from build123d import *

# Parameters (mm, degrees)
SKETCH1_W           = 168
SKETCH1_H           = 48
SKETCH1_W_2         = 42
SKETCH1_H_2         = 42
SKETCH1_W_3         = 72
BOSS_EXTRUDE1_DEPTH = 10
SKETCH2_W           = 18
SKETCH2_H           = 10
CUT_EXTRUDE1_DEPTH  = 10
SKETCH3_W           = 42
SKETCH3_H           = 42
SKETCH3_W_2         = 32
SKETCH3_H_2         = 32
BOSS_EXTRUDE2_DEPTH = 7
BOSS_EXTRUDE3_DEPTH = 7
FILLET1_R           = 10
SKETCH6_W           = 18
SKETCH6_H           = 7
BOSS_EXTRUDE4_DEPTH = 3


with BuildPart() as part:
    # Sketch1 → Boss-Extrude1 (new body)
    with BuildSketch(Plane(origin=(0, 0, 0), x_dir=(1, 0, 0), z_dir=(0, 1, 0))):
        with Locations((-81, 21)):
            Rectangle(SKETCH1_W, SKETCH1_H)
        with Locations((-141, 21)):
            Rectangle(SKETCH1_W_2, SKETCH1_H_2, mode=Mode.SUBTRACT)
        with Locations((-21, 21)):
            Rectangle(SKETCH1_W_2, SKETCH1_H_2, mode=Mode.SUBTRACT)
        with Locations((-81, 21)):
            Rectangle(SKETCH1_W_3, SKETCH1_H_2, mode=Mode.SUBTRACT)
    extrude(amount=BOSS_EXTRUDE1_DEPTH)

    # Sketch2 → Cut-Extrude1 (cut)
    with BuildSketch(Plane(origin=(0, 0, -45), x_dir=(-1, 0, 0), z_dir=(0, 0, -1))):
        with Locations((21, 5)):
            Rectangle(SKETCH2_W, SKETCH2_H)
        with Locations((141, 5)):
            Rectangle(SKETCH2_W, SKETCH2_H)
    extrude(amount=-CUT_EXTRUDE1_DEPTH, mode=Mode.SUBTRACT)

    # Sketch3 → Boss-Extrude2 (add)
    with BuildSketch(Plane.XZ):
        with Locations((-21, -21)):
            Rectangle(SKETCH3_W, SKETCH3_H)
        with Locations((-21, -21)):
            Rectangle(SKETCH3_W_2, SKETCH3_H_2, mode=Mode.SUBTRACT)
    extrude(amount=-BOSS_EXTRUDE2_DEPTH)

    # Sketch4 → Boss-Extrude3 (add)
    with BuildSketch(Plane(origin=(0, 10, 0), x_dir=(1, 0, 0), z_dir=(0, 1, 0))):
        Polygon((-42, 42), (-30, 42), (-30, 45), (-42, 45), (-45, 45), (-45, 42), (-45, 0), (-45, -3), (-42, -3), (3, -3), (3, 0), (3, 42), (3, 45), (0, 45), (-12, 45), (-12, 42), (0, 42), (0, 0), (-42, 0), align=None)
    extrude(amount=BOSS_EXTRUDE3_DEPTH)

    # Fillet1
    fillet1_edges = [part.edges().sort_by_distance(p)[0] for p in [
        (-117, 5, -42),
        (-117, 5, 0),
        (-45, 5, 0),
        (-45, 5, -42),
    ]]
    fillet(fillet1_edges, radius=FILLET1_R)

    # Sketch6 → Boss-Extrude4 (add)
    with BuildSketch(Plane(origin=(0, 0, -42), x_dir=(-1, 0, 0), z_dir=(0, 0, -1))):
        with Locations((21, 3.5)):
            Rectangle(SKETCH6_W, SKETCH6_H)
    extrude(amount=BOSS_EXTRUDE4_DEPTH)


solid = part.part
Verification items for the finished model (mm, model axes). A direction names the side the tool comes from. Round coordinates to 2 decimals unless told otherwise and drop trailing zeros. Loops run counter-clockwise (first coordinate to the right, second up) from the corner with the lowest first, then second, coordinate; pieces in that order, holes last. Notation, with made-up numbers: (66, 21.5) - (110, 21.5) arc R6 ccw to (110, 30.5) - close; hole circle Ø5 at (1.25, 39.25). An arc over 180 degrees is marked (long way). Write item = value, one per line.
Q1. Sectioned sample at D-D on z = -39.5. Record the boundary of the cut face in (x, y).
Here are the results:
outline = (-165, 0) - (-162, 0) - (-162, 10) - (-165, 10) - close; (-120, 0) - (-113.61, 0) - (-113.61, 10) - (-120, 10) - close; (-48.39, 0) - (3, 0) - (3, 17) - (0, 17) - (0, 7) - (-42, 7) - (-42, 17) - (-45, 17) - (-45, 10) - (-48.39, 10) - close
Q2. Tool access check on faces 4 (the flat face through (0, 12, -21)), 5 (the flat face through (-30, 12, -43)), 6 (the flat face through (-150, 5, -44)), 7 (the flat face through (-43, 0, -19)), 8 (the flat face through (-21, 3, -37)). Record the directions out of +Z, -Z, +X, -X, +Y, -Y that give a thin tool (end or side, any length) a straight path to the whole face; none if there is none.
Here are the results:
face_4 = +Y
face_5 = -Z, +Y
face_6 = -Z, +Y, -Y
face_7 = +Z, -Z, +X, -X, -Y
face_8 = +Y, -Y
Q3. Sectioned sample at C-C on y = 5.25. Record the boundary of the cut face in (x, z).
Here are the results:
outline = (-165, -45) - (-150, -45) - (-150, -42) - (-162, -42) - (-162, 0) - (-120, 0) - (-120, -42) - (-132, -42) - (-132, -45) - (3, -45) - (3, 3) - (-165, 3) - close; hole (-117, -32) arc R10 ccw to (-107, -42) - (-55, -42) arc R10 ccw to (-45, -32) - (-45, -10) arc R10 ccw to (-55, 0) - (-107, 0) arc R10 ccw to (-117, -10) - close; hole (-37, -37) - (-5, -37) - (-5, -5) - (-37, -5) - close
Q4. Mould release check, pull along X, two halves, no side actions. Record for faces 1 (the flat face through (-64, 6, 3)), 2 (the flat face through (-81, 5, -42)), 3 (the flat face through (3, 8, -21)): +X half, -X half, draft (parallel to the pull), parting line (faces both ways), or undercut.
Here are the results:
face_1 = draft
face_2 = undercut
face_3 = +X half
Q5. Sectioned sample at B-B on x = -25.5. Record the boundary of the cut face in (y, z), plus the area to 3 significant figures.
Here are the results:
outline = (0, -45) - (7, -45) - (7, -37) - (0, -37) - close; (0, -5) - (7, -5) - (7, 0) - (17, 0) - (17, 3) - (0, 3) - close
area = 142 mm^2
Q6. Sectioned sample at A-A on z = -20. Record the boundary of the cut face in (x, y), plus the area to 3 significant figures.
Here are the results:
outline = (-165, 0) - (-162, 0) - (-162, 10) - (-165, 10) - close; (-120, 0) - (-117, 0) - (-117, 10) - (-120, 10) - close; (-45, 0) - (-37, 0) - (-37, 7) - (-42, 7) - (-42, 17) - (-45, 17) - close; (-5, 0) - (3, 0) - (3, 17) - (0, 17) - (0, 7) - (-5, 7) - close
area = 232 mm^2
Q7. Depth check by flat-ended pin: pin 1 (3 mm diameter, centred on x = -149.5, y = 3.5, fed in from -Z). Enter the tip coordinate at first touch or a pass-through.
Here are the results:
pin_1 = -45
Q8. Material ranges on L1, parallel to X at y = 11.75, z = -40.5; L2, parallel to X at y = 1, z = -4.5, recorded low to high.
Here are the results:
L1 = -45 to -42, 0 to 3
L2 = -165 to -162, -120 to -115.35, -46.65 to 3
